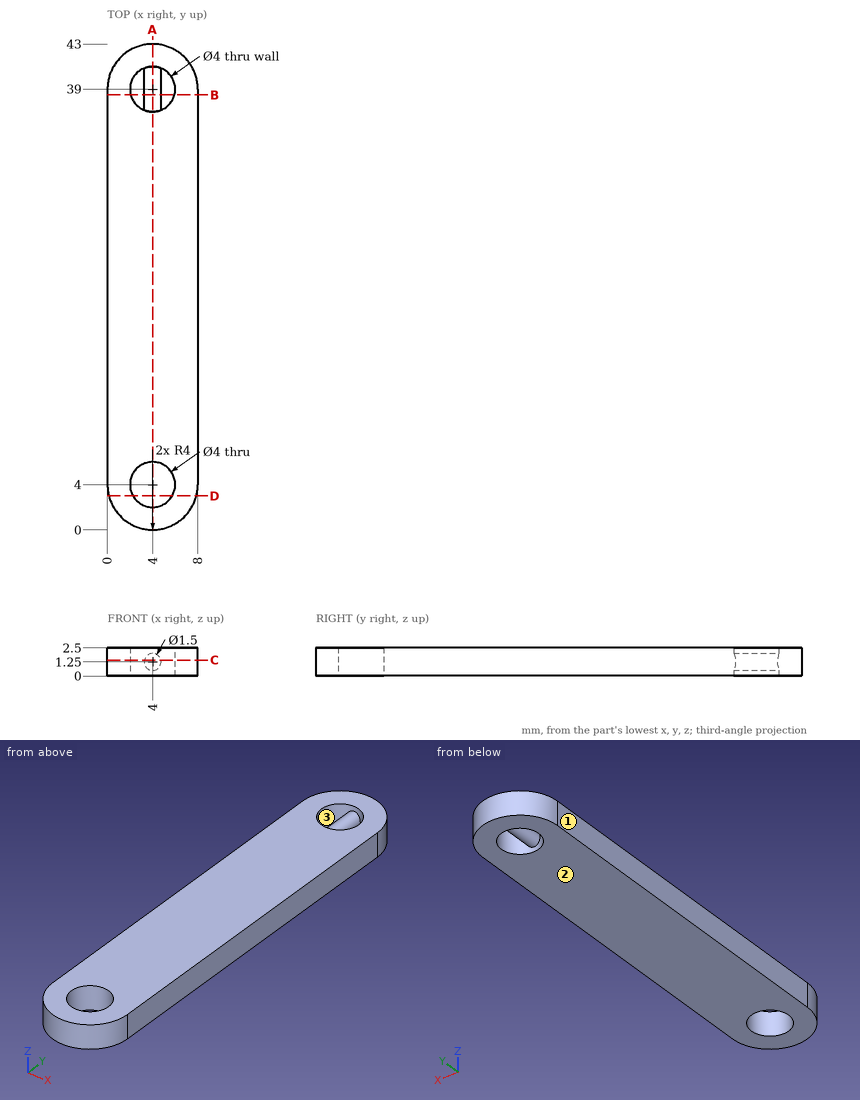
Could you check a few things on this drawing? It's one solid part, dimensions in mm from its lowest x, y, z. Give positions to 0.01 mm unless a question says otherwise; leave off trailing zeros. Write each loop counter-clockwise with the first axis right and the second up, starting at its lowest first coordinate (ties: lowest second). Pieces come first, ordered by that corner, then holes.
(1) Imagine slicing it at B-B, the plane y = 38.5. Write out the boundary of the cut face in (x, z), and give its area (3 significant figures).
Output values:
outline: (0, 0) - (2.06, 0) - (2.06, 2.5) - (0, 2.5) - close; circle Ø1.5 at (4, 1.25); (5.94, 0) - (8, 0) - (8, 2.5) - (5.94, 2.5) - close
area: 12.1 mm2
(2) Will these pins go through, and if not, where does the flat tip stop? pin 1 (1.5 mm diameter, centred on x = 7, z = 0.5, fed in from +Y); pin 2 (1 mm diameter, centred on x = 5, z = 0.5, fed in from +Y).
Output values:
pin 1: stops at y = 42.31
pin 2: stops at y = 42.97
(3) Imagine slicing it at C-C, the plane z = 1.4. Write out the boundary of the cut face in (x, y).
Output values:
outline: (0, 4) arc R4 ccw to (8, 4) - (8, 39) arc R4 ccw to (0, 39) - close; hole circle Ø4 at (4, 4); hole (3.27, 37.14) - (3.27, 40.86) arc R2 ccw to start; hole (4.73, 37.14) arc R2 ccw to (4.73, 40.86) - close
(4) Thinking about a two-plate mould opening in X: for the marked faces 1, 2 and 3, which applies, pulls with the +X half, pulls with the -X half, needs draft (parallel to the pull), parting line crosses it, or undercut?
Output values:
face 1: pulls with the -X half
face 2: needs draft
face 3: undercut
(5) Imagine slicing it at A-A, the plane x = 4. Write out the boundary of the cut face in (y, z), and give its area (3 significant figures).
Output values:
outline: (0, 0) - (2, 0) - (2, 2.5) - (0, 2.5) - close; (6, 0) - (37, 0) - (37, 0.5) - (41, 0.5) - (41, 0) - (43, 0) - (43, 2.5) - (41, 2.5) - (41, 2) - (37, 2) - (37, 2.5) - (6, 2.5) - close
area: 93.5 mm2
(6) If I drill on L1, parallel to Y at x = 4, z = 1.05; L2, parallel to Y at x = 3, z = 1.8; L3, parallel to Y at x = 2.75, z = 1.45, over which ranges is the centre line in solid material (lowest first)?
Output values:
L1: y = 0 to 2, 6 to 43
L2: y = 0.13 to 2.27, 5.73 to 37.27, 40.73 to 42.87
L3: y = 0.2 to 2.44, 5.56 to 37.44, 40.56 to 42.8
(7) Imagine slicing it at D-D, the plane y = 3. Write out the boundary of the cut face in (x, z).
Output values:
outline: (0.13, 0) - (2.27, 0) - (2.27, 2.5) - (0.13, 2.5) - close; (5.73, 0) - (7.87, 0) - (7.87, 2.5) - (5.73, 2.5) - close
